```python
from build123d import *

# Parameters (mm, degrees)
F0_R     = 15
F3_DEPTH = 15


with BuildPart() as f2:
    # F0 (on Front) → F2 (revolve)
    with BuildSketch(Plane.XZ):
        with BuildLine():
            ThreePointArc((24.494897, 12.5), (26.738172, 6.428076), (27.5, 0))
            Line((27.5, 0), (250, 0))
            Line((250, 0), (250, 8))
            Line((250, 8), (225, 8))
            Line((225, 8), (225, 8.5))
            Line((225, 8.5), (205, 8.5))
            Line((205, 8.5), (205, 12.5))
            Line((205, 12.5), (24.494897, 12.5))
        make_face()
    revolve(axis=Axis((125.488594, 0, 0), (1, 0, 0)))

    # F0 (on Front) → F3 (join, symmetric)
    with BuildSketch(Plane.XZ):
        with BuildLine():
            ThreePointArc((24.494897, 12.5), (-26.738172, -6.428076), (27.5, 0))
            ThreePointArc((27.5, 0), (26.738172, 6.428076), (24.494897, 12.5))
        make_face()
        Circle(F0_R, mode=Mode.SUBTRACT)
    extrude(amount=F3_DEPTH, both=True)


solid = f2.part
```
Build history of the part. All positions in model axes, mm. A direction names the side the tool comes from. Round coordinates to 2 decimals unless told otherwise and drop trailing zeros. Write each loop counter-clockwise with the first axis right and the second up, starting at its lowest first coordinate (ties: lowest second). Pieces come first, ordered by that corner, then holes. Notation, with made-up numbers: (-7.5, 81.25) - (43.5, 81.25) arc R22 cw to (43.5, 90.25) - close; hole circle Ø9 at (-2, 19). An arc over 180 degrees is marked (long way). Write each question's results on one line, items separated by ' | '. Start each with the question number.
Item 1: Mould opens along Z. For faces 3 (the face through (205, 8.2, 3)), 4 (the face through (-14.985, 0.21, 0.66)), 5 (the face through (237.32, 7.81, -1.73)) say: pulls with the +Z half, pulls with the -Z half, needs draft (parallel to the pull), parting line crosses it, or undercut.
Item 2: Drop flat-ended pins along their axis: P1, Ø10, axis at x = 34, y = 3.5, coming from the -Z side; P2, Ø2, axis at x = 189.5, y = 3.5, coming from the +Z side; P3, Ø5, axis at x = 74, z = 0, coming from the -Y side. Give the stop position or say it passes through.
Item 3: Saw through at D-D (z = 22). Write the cut outline in (x, y).
Item 4: Saw through at B-B (y = 4). Write the cut outline in (x, z).
Item 5: Which spindle directions (+Z, -Z, +X, -X, +Y, -Y) get a long thin tool onto all of the face, cutting with end or side? Do faces 1 (the face through (12, -15, -12)), 2 (the face through (214.86, -7.167, 4.57)). Say none if no direction does.
Item 6: Wall check: L1, parallel to Z at x = 0, y = -3; L2, parallel to X at y = -1.5, z = -4; L3, parallel to Z at x = 85.5, y = -0.5. Give the ranges that are in metal, low to high. Write a range as [from, to].
Item 7: Saw through at C-C (z = 5.5). Write the cut outline in (x, y).
Item 8: Saw through at A-A (x = 0). Write the cut outline in (y, z).
Results are:
1) face 3: needs draft | face 4: undercut | face 5: parting line crosses it
2) P1: stops at z = -12.5 | P2: stops at z = 12.25 | P3: stops at y = -12.5
3) outline: (-16.5, -15) - (16.5, -15) - (16.5, 15) - (-16.5, 15) - close
4) outline: (24.49, 12.5) arc R27.5 ccw (long way) to (24.82, -11.84) - (205, -11.84) - (205, -7.5) - (225, -7.5) - (225, -6.93) - (250, -6.93) - (250, 6.93) - (225, 6.93) - (225, 7.5) - (205, 7.5) - (205, 11.84) - (24.82, 11.84) arc R27.5 ccw to start; hole circle Ø30 at (0, 0)
5) face 1: +Z, -Z, +X, -X, -Y | face 2: +X
6) L1: z = [-27.5, -15], [15, 27.5] | L2: x = [-27.21, -14.46], [14.46, 250] | L3: z = [-12.49, 12.49]
7) outline: (-26.94, -15) - (-13.96, -15) - (-13.96, 15) - (-26.94, 15) - close; (13.96, -15) - (26.94, -15) - (26.94, -11.22) - (205, -11.22) - (205, -6.48) - (225, -6.48) - (225, -5.81) - (250, -5.81) - (250, 5.81) - (225, 5.81) - (225, 6.48) - (205, 6.48) - (205, 11.22) - (26.94, 11.22) - (26.94, 15) - (13.96, 15) - close
8) outline: (-15, -27.5) - (15, -27.5) - (15, -15) - (-15, -15) - close; (-15, 15) - (15, 15) - (15, 27.5) - (-15, 27.5) - close
